CAD build for the part. Positions are in the model's coordinates, mm. Face numbers are marked on the shaded views. Coordinates: 2 decimals unless noted, no trailing zeros. Order: outer loops, then holes, each group sorted by start corner. A loop starts at its lowest first (then second) coordinate and runs counter-clockwise, first axis right, second up. Notation, with made-up numbers: (-1, 83.25) - (25, 83.25) arc R15 cw to (25, 97.25) - close; hole circle Ø11 at (-17, 12.5). An arc over 180 degrees is marked (long way). Use one line per item in the form item = value.
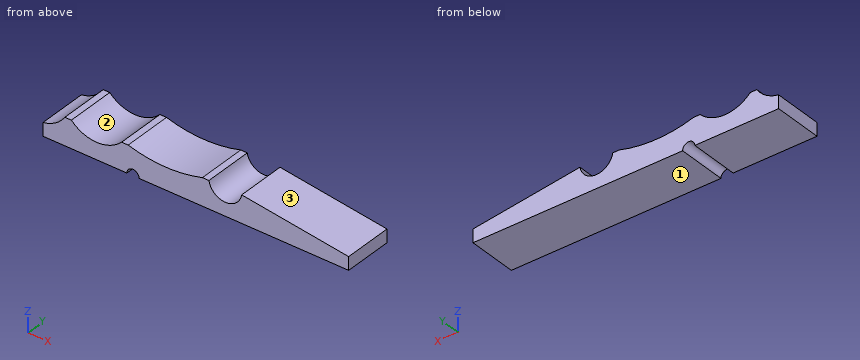
```python
from build123d import *

# Parameters (mm, degrees)
F1_DEPTH = 11.25


with BuildPart() as f1:
    # F0 (on Front) → F1 (new body)
    with BuildSketch(Plane.XZ):
        with BuildLine():
            ThreePointArc((-79.171997, 13.656926), (-81.33179, 11.51529), (-84.171997, 10.426926))
            Line((-84.171997, 10.426926), (-84.171997, 7.426926))
            Line((-84.171997, 7.426926), (-64.971997, 7.426926))
            ThreePointArc((-64.971997, 7.426926), (-63.571997, 8.826926), (-62.171997, 7.426926))
            Line((-62.171997, 7.426926), (-14.171997, 7.426926))
            Line((-14.171997, 7.426926), (-14.171997, 10.426926))
            Line((-14.171997, 10.426926), (-38.671997, 13.656926))
            ThreePointArc((-38.671997, 13.656926), (-42.421997, 10.46775), (-46.171997, 13.656926))
            Line((-46.171997, 13.656926), (-47.671997, 13.656926))
            ThreePointArc((-47.671997, 13.656926), (-56.171997, 12.426926), (-64.671997, 13.656926))
            Line((-64.671997, 13.656926), (-66.171997, 13.656926))
            ThreePointArc((-66.171997, 13.656926), (-71.921997, 11.226926), (-77.671997, 13.656926))
            Line((-77.671997, 13.656926), (-79.171997, 13.656926))
        make_face()
    extrude(amount=F1_DEPTH)


solid = f1.part
```
Item 1: Two-plate mould, pull along X, no slides. Class the marked faces 1, 2 and 3: +X half, -X half, draft (parallel to the pull), parting line (faces both ways), or undercut.
Derived:
face_1 = draft
face_2 = undercut
face_3 = +X half
Item 2: Cut at B-B, the plane z = 8.25. Write the cut outline in (x, y).
Derived:
outline = (-84.17, -11.25) - (-64.7, -11.25) - (-64.7, 0) - (-84.17, 0) - close; (-62.44, -11.25) - (-14.17, -11.25) - (-14.17, 0) - (-62.44, 0) - close
Item 3: Drop a flat-ended pin along its axis: pin 1 (1 mm diameter, centred on y = -5, z = 12.5, fed in from -X). Give the stop position or say it passes through.
Derived:
pin_1 = -80.67
Item 4: Cut at C-C, the plane x = -53.5. Write the cut outline in (y, z), plus the area to 3 significant figures.
Derived:
outline = (-11.25, 7.43) - (0, 7.43) - (0, 12.55) - (-11.25, 12.55) - close
area = 57.6 mm²
Item 5: Cut at D-D, the plane x = -67.5. Write the cut outline in (y, z), plus the area to 3 significant figures.
Derived:
outline = (-11.25, 7.43) - (0, 7.43) - (0, 12.56) - (-11.25, 12.56) - close
area = 57.7 mm²
Item 6: Cut at A-A, the plane y = -6.5. Write the cut outline in (x, z), plus the area to 3 significant figures.
Derived:
outline = (-84.17, 7.43) - (-64.97, 7.43) arc R1.4 cw to (-62.17, 7.43) - (-14.17, 7.43) - (-14.17, 10.43) - (-38.67, 13.66) arc R3.8 cw to (-46.17, 13.66) - (-47.67, 13.66) arc R29.98 cw to (-64.67, 13.66) - (-66.17, 13.66) arc R8.02 cw to (-77.67, 13.66) - (-79.17, 13.66) arc R7.38 cw to (-84.17, 10.43) - close
area = 332 mm²
Item 7: Drill centre lines: line 1 (Z direction, x = -57, y = -2.5); line 2 (X direction, y = -8, z = 8); line 3 (Z direction, x = -57.5, y = -0.5). Where is each one in solid material? Low to high. Write a range as [from, to].
Derived:
line_1 = [7.43, 12.44]
line_2 = [-84.17, -64.85], [-62.29, -14.17]
line_3 = [7.43, 12.46]
